For this review, take the finished solid that the model builds, in its own axes (mm). A direction names the side the tool comes from. Coordinates: 2 decimals unless noted, no trailing zeros. Loops run counter-clockwise (first coordinate to the right, second up) from the corner with the lowest first, then second, coordinate; pieces in that order, holes last. Notation, with made-up numbers: M 58,-22.75 L 104,-22.75 A16 ccw 104,-13.75 Z; hole C -23.75,53.5 d8. An arc over 180 degrees is marked long. Use one line per item in the form item = value.
```python
from build123d import *

# Parameters (mm, degrees)
PAD_DEPTH    = 0.5
SKETCH001_W  = 2
SKETCH001_H  = 100
PAD001_DEPTH = 2
SKETCH002_W  = 18.6
SKETCH002_H  = 12.5
SKETCH002_R  = 2.145
PAD002_DEPTH = 2


with BuildPart() as part:
    # Sketch → Pad (new body, symmetric)
    with BuildSketch(Plane.XY):
        Polygon((-12.731854, 54), (5.868146, 54), (5.868146, -53.999996), (1.568146, -57.999992), (1.568146, -66), (-8.431854, -66), (-8.431854, -57.999992), (-12.731854, -53.999996), align=None)
    extrude(amount=PAD_DEPTH, both=True)

    # Sketch001 (on Face10 of Pad) → Pad001 (join)
    with BuildSketch(Plane.XY.offset(0.5)):
        with Locations((-3.431854, 0)):
            Rectangle(SKETCH001_W, SKETCH001_H)
    extrude(amount=PAD001_DEPTH)

    # Sketch002 (on Face1 of Pad001) → Pad002 (join)
    with BuildSketch(Plane(origin=(0, 54, 0), x_dir=(-1, 0, 0), z_dir=(0, 1, 0))):
        with Locations((6.431854, 5.75)):
            Rectangle(SKETCH002_W, SKETCH002_H)
        with Locations((10.876855, 5.355)):
            Circle(SKETCH002_R, mode=Mode.SUBTRACT)
    extrude(amount=PAD002_DEPTH)


solid = part.part
```
1. Consider section D-D on x = -5.5. Write out the cut boundary in (y, z), plus the area to 3 significant figures.
Computed values:
outline = M -66,-0.5 L 56,-0.5 L 56,12 L 54,12 L 54,0.5 L -66,0.5 Z
area = 145 mm2
2. Consider section B-B on y = -48.5. Write out the cut boundary in (x, z).
Computed values:
outline = M -12.73,-0.5 L 5.87,-0.5 L 5.87,0.5 L -2.43,0.5 L -2.43,2.5 L -4.43,2.5 L -4.43,0.5 L -12.73,0.5 Z
3. Tool access review of faces 1 (the face through (-3, 50, 1)), 2 (the face through (-3, 1, 2.5)), 3 (the face through (-2.432, -1, 1)): name each direction out of +Z, -Z, +X, -X, +Y, -Y from which nothing blocks a thin tool from reaching the whole face with its end or side.
Computed values:
face_1 = +Z, +X, -X
face_2 = +Z, +X, -X, -Y
face_3 = +Z, +X, -Y
4. Consider section A-A on x = -10.5. Write out the cut boundary in (y, z).
Computed values:
outline = M -56.08,-0.5 L 56,-0.5 L 56,3.24 L 54,3.24 L 54,0.5 L -56.08,0.5 Z; M 54,7.47 L 56,7.47 L 56,12 L 54,12 Z
5. Draft analysis for pull direction X (two halves, no side actions). For faces 4 (the face through (2.868, 55, 6)), 5 (the face through (-3, -50, 1)), 6 (the face through (-4.432, -1, 1)), 7 (the face through (-11.867, 54.986, 3.452)), state which applies: +X half, -X half, draft (parallel to the pull), parting line (faces both ways), or undercut.
Computed values:
face_4 = +X half
face_5 = draft
face_6 = -X half
face_7 = undercut
6. Consider section C-C on z = 8.5. Write out the cut boundary in (x, y), plus the area to 3 significant figures.
Computed values:
outline = M -15.73,54 L 2.87,54 L 2.87,56 L -15.73,56 Z
area = 37.2 mm2
7. Wall thickness on line 1 along Y through (x, z) = (-13.5, 10); line 2 along Z through (x, y) = (-11.25, -54.5); line 3 along X through (y, z) = (6, 2): over which ranges is each line inside the solid? List them lowest first. Write a range as from..to.
Computed values:
line_1 = 54..56
line_2 = -0.5..0.5
line_3 = -4.43..-2.43
8. For pin 1 Ø0.6 at (x, y) = (-3.5, 19) entering from +Z; pin 2 Ø1.1 at (y, z) = (-60.5, 0) entering from +X; pin 3 Ø5 at (y, z) = (43, 4) entering from +X, all flat-tipped, find the tip position at first contact; note any pin that passes through.
Computed values:
pin_1 = 2.5
pin_2 = 1.57
pin_3 = -2.43
